Solid Edge part; units mm, degrees
sketch "Sketch1" plane through (0, 0, 0) normal (0, 0, 1) x (1, 0, 0)
  arc A0 (427.7716, 359.5398) -> (0.4572, 558.7998) centre (0, 0) ccw
  line L0 (0.4572, 558.7998) -> (0.4572, 1930.3999)
  arc A1 (1478.4783, 1241.1874) -> (0.4572, 1930.3999) centre (0, 0) ccw
  line L1 (427.7716, 359.5398) -> (1478.4783, 1241.1874)
extrude "Protrusion1" add sketch "Sketch1" against normal blind 6.35
sketch "Sketch2" plane through (739.4677, 1144.9699, 0) normal (0, 0, 1) x (-0.766, -0.6428, 0)
  circle A0 centre (174.4469, -124.2136) radius 409.575
  circle A1 centre (174.4469, -124.2136) radius 403.225
extrude "ExtrudedProtrusion_4" add sketch "Sketch2" along normal blind 12.7
chamfer "Chamfer_1" distance 12.7 angle 45 1 edges at (839.7433, 1391.2604, 12.7)
sketch "Sketch3" plane through (739.4677, 1144.9699, -6.35) normal (0, 0, -1) x (-0.766, -0.6428, 0)
  circle A0 centre (174.4469, 124.2136) radius 409.575
  circle A1 centre (174.4469, 124.2136) radius 403.225
extrude "ExtrudedProtrusion_7" add sketch "Sketch3" along normal blind 12.7
chamfer "Chamfer_4" distance 12.7 angle 45 1 edges at (839.7433, 1391.2604, -19.05)
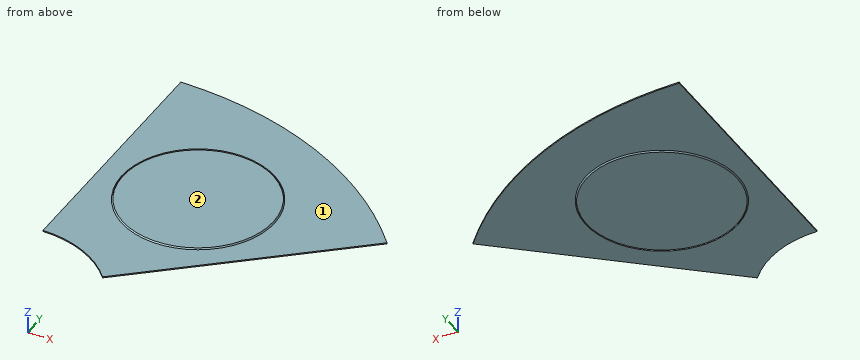
Geometry: final body of the model. Coordinates: model frame, mm. Face numbers are marked on the shaded views. Round coordinates to 2 decimals unless told otherwise and drop trailing zeros. Order: outer loops, then holes, each group sorted by start corner. A loop starts at its lowest first (then second) coordinate and runs counter-clockwise, first axis right, second up. Notation, with made-up numbers: (-35.75, -24) - (-0.75, -24) arc R22 cw to (-0.75, 7) - close; hole circle Ø9 at (-21.5, 5). An arc over 180 degrees is marked (long way). Use CSV: the item, a comma, the result in double quotes. Start each with the question number.
Q1. Mould query, pull axis Y, two halves, no side actions, for the marked faces 1 and 2. Classes: +Y half, -Y half, draft (parallel to the pull), parting line (faces both ways), or undercut.
Q2. Section query A-A (z = -3). Return loops of the section in (x, y).
Q3. First-contact query: pin 1 (10 mm diameter, centred on y = 1181, z = -9, fed in from -X); pin 2 (5 mm diameter, centred on y = 1135, z = -8, fed in from +X); pin 3 (1.5 mm diameter, centred on x = 739.5, y = 1268, fed in from +Z); pin 4 (10 mm diameter, centred on x = 501, z = -10.5, fed in from +Y). Flat tips, straight axial feed; report the tip coordinate or a pass-through.
Q4. Material intervals for line 1 along Z through (x, y) = (881, 1046); line 2 along X through (y, z) = (909, -8.75); line 3 along Y through (x, z) = (593.5, 5.5), sorted ascending. Write a range as from..to.
Q5. Section query B-B (y = 1788). Return loops of the section in (x, z), and give its area (3 significant figures).
Result set:
1,face 1,"draft"
1,face 2,"undercut"
2,outline,"(0.46, 558.8) arc R558.8 cw to (427.77, 359.54) - (1478.48, 1241.19) arc R1930.4 ccw to (0.46, 1930.4) - close"
3,pin 1,"stops at x = 0.46"
3,pin 2,"stops at x = 1354.17"
3,pin 3,"stops at z = 0"
3,pin 4,"stops at y = 1865"
4,line 1,"z = -6.35..0"
4,line 2,"x = 182.72..187.42, 864.57..869.26"
4,line 3,"y = 729.6..730.46, 1525.52..1526.39"
5,outline,"(0.46, -6.35) - (727.67, -6.35) - (727.67, 0) - (0.46, 0) - close"
5,area,"4,620 mm2"
